Geometry check sheet. Reference: the model listing, model coordinates, mm. A direction names the side the tool comes from. Coordinates: 2 decimals unless noted, no trailing zeros. Loops run counter-clockwise (first coordinate to the right, second up) from the corner with the lowest first, then second, coordinate; pieces in that order, holes last. Notation, with made-up numbers: (45.25, -27.5) - (84.25, -27.5) arc R21 ccw to (84.25, -4.5) - close; hole circle Ø7 at (79, 65.5). An arc over 180 degrees is marked (long way). Write each question's results on one line, items separated by ' | '. Start each with the question number.
(1) Go/stop test with flat-tipped pins: pin 1 Ø10 at (y, z) = (36.5, 21) entering from -X; pin 2 Ø6 at (x, z) = (9, 25) entering from -Y; pin 3 Ø3 at (x, y) = (12.5, 12) entering from +Z; pin 4 Ø6 at (x, z) = (19.5, 23) entering from -Y. Record where each tip stops, or that it passes through.
(2) Sectioned sample at C-C (z = 14). Enter the section's corners in (x, y), plus the area to 3 significant figures.
(3) Mould release check, pull along Y, two halves, no side actions. Record for faces 6 (the face through (0, -56, 6)), 7 (the face through (-16, 45, 41)), 8 (the face through (6, 40, 19)): pulls with the +Y half, pulls with the -Y half, needs draft (parallel to the pull), parting line crosses it, or undercut.
(4) Sectioned sample at D-D (x = 0). Enter the section's corners in (y, z).
(5) Sectioned sample at B-B (y = -42). Enter the section's corners in (x, z).
(6) Access from +Z, -Z, +X, -X, +Y, -Y to the whole of each face (thin tool, end or side, straight path). Record for faces 1 (the face through (-8, -46, 5)), 2 (the face through (0, -42, 11)), 3 (the face through (0, -38, 0)), 4 (the face through (-6.489, 46, 33)), 5 (the face through (0, 34, 11)).
(7) Material ranges on probe 1 along X at (y, z) = (-42, 4); probe 2 along Y at (x, z) = (-11, 8); probe 3 along Y at (x, z) = (-19.5, 13), recorded low to high.
(8) Sectioned sample at A-A (x = 11). Enter the section's corners in (y, z).
from build123d import *

# Parameters (mm, degrees)
F0_W     = 11
F0_H     = 30
F1_DEPTH = 25
F4_DEPTH = 11
F5_R     = 5
F6_DEPTH = 11


with BuildPart() as f1:
    # F0 (on Right) → F1 (new body)
    with BuildSketch(Plane.YZ):
        with Locations((45.5, 26)):
            Rectangle(F0_W, F0_H)
        with BuildLine():
            ThreePointArc((27.910571, 11), (29.473014, 5.598342), (30, 0))
            Line((30, 0), (51, 0))
            Line((51, 0), (51, 11))
            Line((51, 11), (40, 11))
            Line((40, 11), (27.910571, 11))
        make_face()
        with BuildLine():
            ThreePointArc((-15.491933, 11), (0, 19), (15.491933, 11))
            Line((15.491933, 11), (27.910571, 11))
            ThreePointArc((27.910571, 11), (0, 30), (-27.910571, 11))
            Line((-27.910571, 11), (-15.491933, 11))
        make_face()
        with BuildLine():
            Line((-30, 0), (-19, 0))
            ThreePointArc((-19, 0), (-18.10175, 5.772922), (-15.491933, 11))
            Line((-15.491933, 11), (-27.910571, 11))
            ThreePointArc((-27.910571, 11), (-29.473014, 5.598342), (-30, 0))
        make_face()
        with BuildLine():
            ThreePointArc((15.491933, 11), (18.10175, 5.772922), (19, 0))
            Line((19, 0), (30, 0))
            ThreePointArc((30, 0), (29.473014, 5.598342), (27.910571, 11))
            Line((27.910571, 11), (15.491933, 11))
        make_face()
        with BuildLine():
            Line((-56, 0), (-30, 0))
            ThreePointArc((-30, 0), (-29.473014, 5.598342), (-27.910571, 11))
            Line((-27.910571, 11), (-56, 11))
            Line((-56, 11), (-56, 0))
        make_face()
    extrude(amount=F1_DEPTH)

    # F2: F1 across face


with BuildPart() as f1_1:
    add(f1.part)
    add(f1.part.mirror(Plane(origin=(0, 7.065058, 14.616271), x_dir=(0, 1, 0), z_dir=(-1, 0, 0))))

    # F3 (on face) → F4 (cut)
    with BuildSketch(Plane(origin=(0, 51, 0), x_dir=(-1, 0, 0), z_dir=(0, 1, 0))):
        with BuildLine():
            ThreePointArc((-6.42497, 25.984765), (-0.49381, 18.518785), (6.5, 25))
            ThreePointArc((6.5, 25), (6.497197, 25.190868), (6.488791, 25.381571))
            ThreePointArc((6.488791, 25.381571), (0.303281, 31.492921), (-6.42497, 25.984765))
        make_face()
        with BuildLine():
            ThreePointArc((-6.42497, 25.984765), (0.303281, 31.492921), (6.488791, 25.381571))
            Line((6.488791, 25.381571), (6.488791, 41))
            Line((6.488791, 41), (-6.42497, 41))
            Line((-6.42497, 41), (-6.42497, 25.984765))
        make_face()
    extrude(amount=-F4_DEPTH, mode=Mode.SUBTRACT)

    # F5 (on face) → F6 (cut)
    with BuildSketch(Plane(origin=(0, 0, 0), x_dir=(1, 0, 0), z_dir=(0, 0, -1))):
        with Locations((-11, 42)):
            Circle(F5_R)
        with Locations((11, 42)):
            Circle(F5_R)
    extrude(amount=-F6_DEPTH, mode=Mode.SUBTRACT)


solid = f1_1.part
Outcome:
1) pin 1: stops at x = -25 | pin 2: stops at y = -20.4 | pin 3: stops at z = 28.1 | pin 4: stops at y = -22.36
2) outline: (-25, -26.53) - (25, -26.53) - (25, -12.85) - (-25, -12.85) - close; (-25, 12.85) - (25, 12.85) - (25, 26.53) - (-25, 26.53) - close; (-25, 40) - (25, 40) - (25, 51) - (-25, 51) - close | area: 1,920 mm2
3) face 6: pulls with the -Y half | face 7: needs draft | face 8: undercut
4) outline: (-56, 0) - (-19, 0) arc R19 cw to (-15.49, 11) arc R19 cw to (15.49, 11) arc R19 cw to (19, 0) - (51, 0) - (51, 18.5) - (40, 18.5) - (40, 11) - (27.91, 11) arc R30 ccw to (-27.91, 11) - (-56, 11) - close
5) outline: (-25, 0) - (-16, 0) - (-16, 11) - (-25, 11) - close; (-6, 0) - (6, 0) - (6, 11) - (-6, 11) - close; (16, 0) - (25, 0) - (25, 11) - (16, 11) - close
6) face 1: +Z, -Z | face 2: +Z, +X, -X, -Y | face 3: -Z, +X, -X, +Y, -Y | face 4: +Z, +Y | face 5: +Z, +X, -X
7) probe 1: x = -25 to -16, -6 to 6, 16 to 25 | probe 2: y = -56 to -47, -37 to -17.23, 17.23 to 51 | probe 3: y = -27.04 to -13.86, 13.86 to 27.04, 40 to 51
8) outline: (-56, 0) - (-47, 0) - (-47, 11) - (-56, 11) - close; (-37, 0) - (-19, 0) arc R19 cw to (-15.49, 11) arc R19 cw to (15.49, 11) arc R19 cw to (19, 0) - (51, 0) - (51, 41) - (40, 41) - (40, 11) - (27.91, 11) arc R30 ccw to (-27.91, 11) - (-37, 11) - close
